Autodesk Inventor part; units mm, degrees
ref_plane "Work Plane1" through (-4.7625, 3.81, 0) normal (0, -1, 0) x (1, 0, 0)
ref_plane "YZ Plane" through (0, 0, 0) normal (1, 0, 0) x (0, 1, 0)
ref_plane "XZ Plane" through (0, 0, 0) normal (0, 1, 0) x (-1, 0, 0)
sketch "Sketch1" plane through (0, 0, 0) normal (0, 0, 1) x (1, 0, 0)
  line L0 (0, 0) -> (-4.7625, 0)
  line L1 (-4.7625, 0) -> (-4.7625, 17.646)
  line L2 (0, 17.646) -> (0, 0)
  line L3 (-20.447, 21.837) -> (9.525, 21.837)
  line L4 (9.525, 21.837) -> (9.525, 17.646)
  line L5 (-20.447, 17.646) -> (-20.447, 21.837)
  line L6 (9.525, 17.646) -> (0, 17.646)
  line L7 (-4.7625, 17.646) -> (-20.447, 17.646)
  point P0 (-2.3813, 0)
  dimension "d3" = 4.7625
  dimension "d4" = 4.191
  dimension "d5" = 29.972
  dimension "d6" = 21.837
  dimension "d8" = 9.525
extrude "Extrusion1" add sketch "Sketch1" along normal blind 76.2
sketch "Sketch2" plane through (-4.7625, 0, 0) normal (0, -1, 0) x (1, 0, 0)
  line L0 (0, 0) -> (4.7625, 0)
  line L1 (4.7625, 0) -> (4.7625, 76.2)
  line L2 (0, 76.2) -> (4.7625, 76.2)
  line L3 (0, 0) -> (0, 76.2)
  line L4 (0, 76.2) -> (4.7625, 76.2)
  circle A0 centre (2.2225, 62.2875) radius 2.2
  circle A1 centre (2.2225, 14.2875) radius 2.2
  circle A2 centre (2.2225, 14.2875) radius 1.143
  circle A3 centre (2.2225, 62.2875) radius 1.143
  point P0 (2.3813, 76.2)
  dimension "d52" = 2.286
  dimension "d53" = 2.286
chamfer "Chamfer1" distance 3.175 angle 45 2 edges at (-4.7625, 17.646, 38.1) (0, 17.646, 38.1)
extrude "Extrusion2" cut sketch "Sketch2" against normal blind 6.35 contours A2 | A3
ref_plane "Work Plane1" through (-4.7625, 3.81, 0) normal (0, -1, 0) x (1, 0, 0)
sketch "Sketch3" plane through (-4.7625, 3.81, 0) normal (0, -1, 0) x (1, 0, 0)
  circle A0 centre (2.2225, 62.2875) radius 1.016
  line L0 (4.7625, 60.2555) -> (1.0493, 60.2555)
  line L1 (1.0493, 60.2555) -> (-0.1239, 62.2875)
  line L2 (-0.1239, 62.2875) -> (1.0493, 64.3195)
  line L3 (1.0493, 64.3195) -> (4.7625, 64.3195)
  circle A1 centre (2.2225, 14.2875) radius 1.016
  line L4 (4.7625, 12.2555) -> (1.0493, 12.2555)
  line L5 (1.0493, 12.2555) -> (-0.1239, 14.2875)
  line L6 (-0.1239, 14.2875) -> (1.0493, 16.3195)
  line L7 (1.0493, 16.3195) -> (4.7625, 16.3195)
  line L8 (4.7625, 76.2) -> (4.7625, 0)
  circle A2 centre (2.2225, 14.2875) radius 1.143
  circle A3 centre (2.2225, 62.2875) radius 1.143
  dimension "d21" = 4.064
  dimension "d22" = 4.064
extrude "Extrusion3" cut sketch "Sketch3" against normal mid plane 1.5875 contours L0 L1 L2 L3 L8 | L8 L4 L5 L6 L7 | A1 | A2 | A3
sketch "Sketch5" plane through (-20.447, 17.646, 0) normal (0, -1, 0) x (1, 0, 0)
  circle A0 centre (3.907, 72.5295) radius 1
  circle A1 centre (26.907, 72.5295) radius 1
  circle A2 centre (26.907, 4.0455) radius 1
  circle A3 centre (3.907, 4.0455) radius 1
  point P0 (20.447, 0)
hole "Hole1" at (-16.54, 17.646, 72.5295) at (6.46, 17.646, 72.5295) at (6.46, 17.646, 4.0455) at (-16.54, 17.646, 4.0455) direction (0, 1, 0) diameter 2.286 depth 25.4 tip angle 118 counterbore diameter 4.064 counterbore depth 1.524
sketch "Sketch6" plane through (0, 0, 76.2) normal (0, 0, 1) x (1, 0, 0)
  line L0 (3.175, 17.646) -> (9.525, 17.646)
  line L1 (9.525, 17.646) -> (9.525, 21.837)
  line L2 (9.525, 21.837) -> (-20.447, 21.837)
  line L3 (-20.447, 21.837) -> (-20.447, 17.646)
  line L4 (-20.447, 17.646) -> (-7.9375, 17.646)
  line L5 (-4.7625, 14.471) -> (-7.9375, 17.646)
  line L6 (-4.7625, 14.471) -> (-4.7625, 0)
  line L7 (-4.7625, 0) -> (0, 0)
  line L8 (0, 0) -> (0, 14.471)
  line L9 (3.175, 17.646) -> (0, 14.471)
  line L10 (3.175, 17.646) -> (9.525, 17.646)
  line L11 (-7.9375, 17.646) -> (3.175, 17.646)
extrude "Extrusion5" cut sketch "Sketch6" against normal blind 9.525 contours L9 L8 L7 L6 L5 L11
sketch "Sketch7" plane through (0, 0, 0) normal (0, 0, -1) x (-1, 0, 0)
  line L0 (0, 14.471) -> (-3.175, 17.646)
  line L1 (0, 0) -> (0, 14.471)
  line L2 (4.7625, 0) -> (0, 0)
  line L3 (4.7625, 14.471) -> (4.7625, 0)
  line L4 (7.9375, 17.646) -> (4.7625, 14.471)
  line L5 (20.447, 17.646) -> (7.9375, 17.646)
  line L6 (20.447, 21.837) -> (20.447, 17.646)
  line L7 (-9.525, 21.837) -> (20.447, 21.837)
  line L8 (-9.525, 17.646) -> (-9.525, 21.837)
  line L9 (-3.175, 17.646) -> (-9.525, 17.646)
  line L10 (-3.175, 17.646) -> (8.255, 17.646)
  line L11 (20.447, 17.646) -> (-9.525, 17.646)
extrude "Extrusion6" cut sketch "Sketch7" against normal blind 9.525 contours L0 L10 L4 L3 L2 L1
chamfer "Chamfer2" distance 3.175 angle 45 2 edges at (-2.3813, 17.646, 9.525) (-2.3813, 17.646, 66.675)
properties part number "PCB BRACE"
Source: CAD feature listing. Evaluate the final solid. Frame: model axes, mm. A direction names the side the tool comes from. Coordinates: 2 decimals unless noted, no trailing zeros. Loops run counter-clockwise (first coordinate to the right, second up) from the corner with the lowest first, then second, coordinate; pieces in that order, holes last. Notation, with made-up numbers: M 11.5,-0.5 L 38.5,-0.5 A21 ccw 38.5,17.5 Z; hole C 48,-13.75 d6. An arc over 180 degrees is marked long. Use CSV: the item, a comma, the result in double quotes.
(1) Cut plane B-B on z = 40.5. Return loops of the section in (x, y) (1 decimal), and give its area (3 significant figures).
Answers follow:
outline,"M -20.4,17.6 L -7.9,17.6 L -4.8,14.5 L -4.8,0 L 0,0 L 0,14.5 L 3.2,17.6 L 9.5,17.6 L 9.5,21.8 L -20.4,21.8 Z"
area,"220 mm²"
(2) Contact query for flat-ended pins moving along their axis: pin 1 (4 mm diameter, centred on x = -2, y = 6.5, fed in from +Z) (3 decimals); pin 2 (5.5 mm diameter, centred on x = -16.54, z = 4.05, fed in from -Y); pin 3 (3 mm diameter, centred on y = 9.5, z = 49, fed in from -X). Output: stop coordinate, or through.
Answers follow:
pin 1,"z = 66.675"
pin 2,"y = 17.65"
pin 3,"x = -4.76"
(3) Draft query along Y for faces 1 (the face through (0, 7, 38)), 2 (the face through (-6.37, 16.08, 38.54)), 3 (the face through (-2, 4, 16.32)). Return one class per face: pulls with the +Y half, pulls with the -Y half, needs draft (parallel to the pull), parting line crosses it, or undercut.
Answers follow:
face 1,"needs draft"
face 2,"pulls with the -Y half"
face 3,"undercut"
(4) Cut plane A-A on x = 6.46. Return loops of the section in (y, z), and give its area (3 significant figures).
Answers follow:
outline,"M 17.65,0 L 21.84,0 L 21.84,2.9 L 19.17,2.9 L 19.17,2.01 L 17.65,2.01 Z; M 17.65,6.08 L 19.17,6.08 L 19.17,5.19 L 21.84,5.19 L 21.84,71.39 L 19.17,71.39 L 19.17,70.5 L 17.65,70.5 Z; M 17.65,74.56 L 19.17,74.56 L 19.17,73.67 L 21.84,73.67 L 21.84,76.2 L 17.65,76.2 Z"
area,"295 mm²"
(5) Line query: line 1 (Z direction, x = -2.54, y = 5.1) (1 decimal); line 2 (Z direction, x = 6.46, y = 18.25); line 3 (Y direction, x = -1, z = 64). Output: solid intervals per line, ascending. Write a range as [from, to].
Answers follow:
line 1,"[9.5, 13.1], [15.4, 61.1], [63.4, 66.7]"
line 2,"[0, 2.01], [6.08, 70.5], [74.56, 76.2]"
line 3,"[0, 3.02], [4.6, 21.84]"
(6) Cut plane D-D on x = -7. Return loops of the section in (y, z).
Answers follow:
outline,"M 16.71,7.29 L 17.65,6.35 L 17.65,0 L 21.84,0 L 21.84,76.2 L 17.65,76.2 L 17.65,69.85 L 16.71,68.91 Z"
(7) Reachability of faces 4 (the face through (-1, 4.604, 14)), 5 (the face through (-4.762, 7, 38)), 6 (the face through (6, 19.17, 71)) from +Z, -Z, +X, -X, +Y, -Y: full face, straight path, thin tool, end or side. Return the list, or none.
Answers follow:
face 4,"+X"
face 5,"+Z, -Z, -X, -Y"
face 6,"-Y"
